Check sheet for the modelled part. Datum: model origin and axes. Units: mm. A direction names the side the tool comes from. Give positions to 0.01 mm unless a question says otherwise; leave off trailing zeros. Write each loop counter-clockwise with the first axis right and the second up, starting at its lowest first coordinate (ties: lowest second). Pieces come first, ordered by that corner, then holes. Notation, with made-up numbers: (-14, 68) -> (34, 68) arc R20 ccw to (34, 102) -> close; hole circle Ø10 at (18.25, -26.5). An arc over 180 degrees is marked (long way). Write each question's results on one line, items separated by ' | '. Start each with the question number.
```python
from build123d import *

# Parameters (mm, degrees)
CHAMFER1_SIZE      = 0.4
FILLET1_R          = 0.4
CUT_EXTRUDE1_DEPTH = 1.91


with BuildPart() as part:
    # Sketch1 → Revolve1 (revolve)
    with BuildSketch(Plane.XY, mode=Mode.PRIVATE) as revolve1_sk:
        Polygon((0, 0), (0, 3.82), (3.39, 3.82), (3.39, 0), (2, 0), (2, -20), (0, -20), align=None)
    revolve(revolve1_sk.sketch.rotate(Axis((0, 3.82, 0), (0, 1, 0)), 90), axis=Axis((0, 3.82, 0), (0, 1, 0)))

    # Chamfer1
    chamfer1_edges = [part.edges().sort_by_distance(p)[0] for p in [
        (0, -20, 2),
    ]]
    chamfer(chamfer1_edges, length=CHAMFER1_SIZE)

    # Fillet1
    fillet1_edges = [part.edges().sort_by_distance(p)[0] for p in [
        (0, 3.82, 3.39),
    ]]
    fillet(fillet1_edges, radius=FILLET1_R)

    # Sketch2 → Cut-Extrude1 (cut)
    with BuildSketch(Plane(origin=(0, 3.82, 0), x_dir=(1, 0, 0), z_dir=(0, 1, 0))):
        Polygon((0.866025404, -1.5), (1.732050808, 0), (0.866025404, 1.5), (-0.866025404, 1.5), (-1.732050808, 0), (-0.866025404, -1.5), align=None)
    extrude(amount=-CUT_EXTRUDE1_DEPTH, mode=Mode.SUBTRACT)


solid = part.part
```
Item 1: Set-up check for faces 1 (the flat face through (-1.293, 2.878, -0.76)), 2 (the cylindrical face through (2, -10, 0)), 3 (the flat face through (0, -20, 0)): record each of +Z, -Z, +X, -X, +Y, -Y from which the full face is reachable in a straight line by a thin tool's end or side.
Item 2: Thickness scan on probe 1 along Z at (x, y) = (1, -10.5); probe 2 along Y at (x, z) = (2, -1); probe 3 along X at (y, z) = (-10.5, -1.75). Record the ranges inside material, lowest first. Write a range as from..to.
Item 3: Mould release check, pull along Z, two halves, no side actions. Record for faces 4 (the flat face through (0, 0, -2.2)), 5 (the flat face through (1.293, 2.878, 0.76)), 6 (the cylindrical face through (-3.36, 1.69, 0.44)): pulls with the +Z half, pulls with the -Z half, needs draft (parallel to the pull), parting line crosses it, or undercut.
Item 4: Depth check by flat-ended pin: pin 1 Ø4 at (y, z) = (-7.5, 0) entering from -X; pin 2 Ø4 at (y, z) = (-5, 2.5) entering from +X. Enter the tip coordinate at first touch or a pass-through.
Item 5: Section check A-A on x = 0. Record the boundary of the cut face in (y, z).
Item 6: Section check B-B on y = -2.5. Record the boundary of the cut face in (x, z).
Check sheet entries:
1) face 1: +Y | face 2: -Y | face 3: +Z, -Z, +X, -X, -Y
2) probe 1: z = -1.73..1.73 | probe 2: y = 0..3.82 | probe 3: x = -0.97..0.97
3) face 4: needs draft | face 5: undercut | face 6: parting line crosses it
4) pin 1: stops at x = -2 | pin 2: stops at x = 1.94
5) outline: (-20, -1.6) -> (-19.6, -2) -> (0, -2) -> (0, -3.39) -> (3.42, -3.39) arc R0.4 ccw to (3.82, -2.99) -> (3.82, -1.5) -> (1.91, -1.5) -> (1.91, 1.5) -> (3.82, 1.5) -> (3.82, 2.99) arc R0.4 ccw to (3.42, 3.39) -> (0, 3.39) -> (0, 2) -> (-19.6, 2) -> (-20, 1.6) -> close
6) outline: circle Ø4 at (0, 0)
